Geometry: final body of the model. Coordinates: model frame, mm. Face numbers are marked on the shaded views. A direction names the side the tool comes from. Coordinates: 2 decimals unless noted, no trailing zeros. Write each loop counter-clockwise with the first axis right and the second up, starting at its lowest first coordinate (ties: lowest second). Pieces come first, ordered by that corner, then holes. Notation, with made-up numbers: (79, 45.5) - (89, 45.5) arc R22 ccw to (89, 52.5) - close; hole circle Ø1 at (30, 7). An arc over 180 degrees is marked (long way). Answer as a JSON object with one key per item and string values. Group by question number.
Item 1: Line query: line 1 along Z through (x, y) = (12, 10); line 2 along X through (y, z) = (-10.5, 31); line 3 along Y through (x, z) = (43, 7). Output: solid intervals per line, ascending. Write a range as from..to.
Item 2: Section B-B on x = 15. Return loops of the section in (y, z).
Item 3: Section A-A on y = -31. Return loops of the section in (x, z).
Item 4: Set-up query: the marked faces 1, 2 and 3. Return all of +Z, -Z, +X, -X, +Y, -Y with unobstructed straight access to the full face (end or side cutting, diameter ignored); none if empty.
Item 5: First-contact query: pin 1 Ø1 at (x, y) = (-23.5, -36) entering from +Z; pin 2 Ø8 at (x, y) = (15.5, 22.5) entering from +Z; pin 3 Ø15.5 at (x, z) = (8.5, 14.5) entering from -Y. Flat tips, straight axial feed; report the tip coordinate or a pass-through.
Item 6: Section D-D on z = 41. Return loops of the section in (x, y), and give its area (3 significant figures).
Item 7: Section C-C on y = 21.5. Return loops of the section in (x, z), and give its area (3 significant figures).
Item 8: Mould query, pull axis Y, two halves, no side actions, for the marked faces 4, 5 and 6. Classes: pulls with the +Y half, pulls with the -Y half, needs draft (parallel to the pull), parting line crosses it, or undercut.
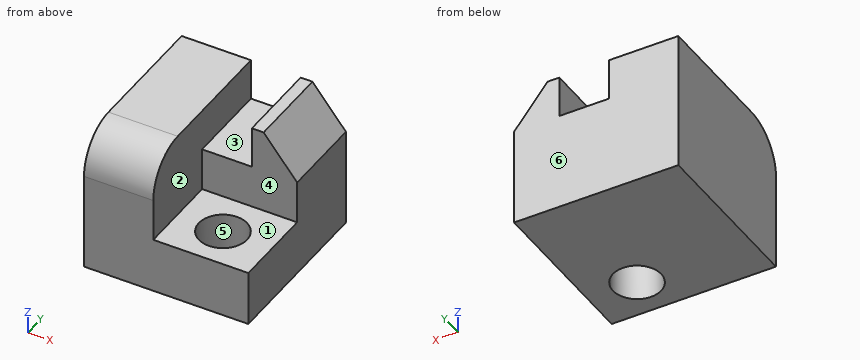
```python
from build123d import *

# Parameters (mm, degrees)
F1_DEPTH = 50.8
F3_DEPTH = 50.8
F4_R     = 25.4
F5_R     = 14.543371
F6_DEPTH = 33.3385


with BuildPart() as f1:
    # F0 (on Front) → F1 (new body, symmetric)
    with BuildSketch(Plane.XZ):
        Polygon((-48.4505, 51.117502), (-48.4505, -33.3375), (50.673001, -33.3375), (50.673001, 26.003249), (30.448252, 51.117502), (23.336248, 51.117502), (23.336248, 26.003249), (-6.6675, 26.003249), (-6.6675, 51.117502), align=None)
    extrude(amount=F1_DEPTH, both=True)

    # F2 (on face) → F3 (cut)
    with BuildSketch(Plane.XZ.offset(50.8)):
        Polygon((23.336248, 26.003249), (-6.6675, 26.003249), (-6.6675, 0), (50.673001, 0), (50.673001, 26.003249), (30.448252, 51.117502), (23.336248, 51.117502), align=None)
    extrude(amount=-F3_DEPTH, mode=Mode.SUBTRACT)

    # F4
    f4_edges = [f1.edges().sort_by_distance(p)[0] for p in [
        (-27.559, -50.8, 51.117502),
    ]]
    fillet(f4_edges, radius=F4_R)

    # F5 (on Top) → F6 (cut, through all)
    with BuildSketch(Plane.XY):
        with Locations((21.113751, -26.2255)):
            Circle(F5_R)
    extrude(amount=-F6_DEPTH, mode=Mode.SUBTRACT)


solid = f1.part
```
Checks:
{
 "1": {"line 1": "-33.34..26", "line 2": "-48.45..-6.67", "line 3": "0..50.8"},
 "2": {"outline": "(-50.8, -33.34) - (-39.42, -33.34) - (-39.42, 0) - (-50.8, 0) - close; (-13.03, -33.34) - (50.8, -33.34) - (50.8, 26) - (0, 26) - (0, 0) - (-13.03, 0) - close"},
 "3": {"outline": "(-48.45, -33.34) - (7.38, -33.34) - (7.38, 0) - (-6.67, 0) - (-6.67, 50.49) - (-48.45, 50.49) - close; (34.85, -33.34) - (50.67, -33.34) - (50.67, 0) - (34.85, 0) - close"},
 "4": {"face 1": "+Z, +X, -Y", "face 2": "+Z, -Y", "face 3": "+Z, +Y, -Y"},
 "5": {"pin 1": "z = 49.02", "pin 2": "z = 26", "pin 3": "y = 0"},
 "6": {"outline": "(-48.45, -45.69) - (-6.67, -45.69) - (-6.67, 50.8) - (-48.45, 50.8) - close; (23.34, 0) - (38.6, 0) - (38.6, 50.8) - (23.34, 50.8) - close", "area": "4,810 mm^2"},
 "7": {"outline": "(-48.45, -33.34) - (50.67, -33.34) - (50.67, 26) - (30.45, 51.12) - (23.34, 51.12) - (23.34, 26) - (-6.67, 26) - (-6.67, 51.12) - (-48.45, 51.12) - close", "area": "7,360 mm^2"},
 "8": {"face 4": "pulls with the -Y half", "face 5": "undercut", "face 6": "pulls with the +Y half"}
}
